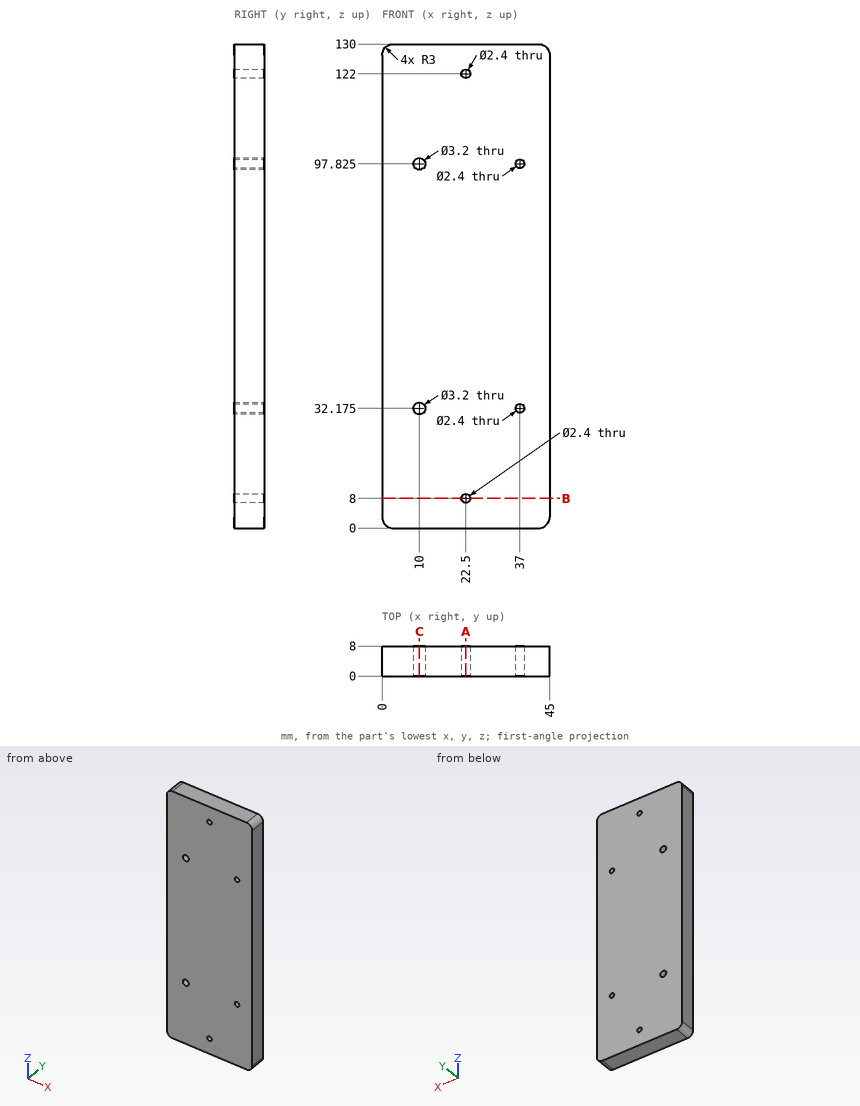
Design review of the part shown in the three views and the two pictorial views. Dimensions are in mm from the part's minimum x, y and z. Round coordinates to 2 decimals unless told otherwise and drop trailing zeros. Order: outer loops, then holes, each group sorted by start corner. A loop starts at its lowest first (then second) coordinate and runs counter-clockwise, first axis right, second up.
(1) Take a section at C-C, the plane x = 10. State the section outline as (y, z) points (3 decimals).
Working result:
outline: (0, 0) - (8, 0) - (8, 30.575) - (0, 30.575) - close; (0, 33.775) - (8, 33.775) - (8, 96.225) - (0, 96.225) - close; (0, 99.425) - (8, 99.425) - (8, 130) - (0, 130) - close
(2) Wall thickness on L1, parallel to Z at x = 23.5, y = 6.25; L2, parallel to X at y = 6, z = 122: over which ranges is each line inside the solid? List them lowest first.
Working result:
L1: z = 0 to 7.34, 8.66 to 121.34, 122.66 to 130
L2: x = 0 to 21.3, 23.7 to 45
(3) Take a section at B-B, the plane z = 8. State the section outline as (x, y) points, plus the area to 3 significant figures.
Working result:
outline: (0, 0) - (21.3, 0) - (21.3, 8) - (0, 8) - close; (23.7, 0) - (45, 0) - (45, 8) - (23.7, 8) - close
area: 341 mm2
(4) For P1, Ø4, axis at x = 40.5, z = 94.5, coming from the -Y side; P2, Ø1.9, axis at x = 10, z = 32.175, coming from the -Y side (1 decimal), all flat-tipped, find the tip position at first contact; note any pin that passes through.
Working result:
P1: stops at y = 0
P2: passes through
(5) Take a section at A-A, the plane x = 22.5. State the section outline as (y, z) points.
Working result:
outline: (0, 0) - (8, 0) - (8, 6.8) - (0, 6.8) - close; (0, 9.2) - (8, 9.2) - (8, 120.8) - (0, 120.8) - close; (0, 123.2) - (8, 123.2) - (8, 130) - (0, 130) - close
